from build123d import *

# Parameters (mm, degrees)
SKETCH1_W           = 50.8
SKETCH1_H           = 25.4
BOSS_EXTRUDE1_DEPTH = 660.4
SKETCH2_R           = 6.35
CUT_EXTRUDE1_DEPTH  = 254


with BuildPart() as part:
    # Sketch1 → Boss-Extrude1 (new body)
    with BuildSketch(Plane.XY):
        with Locations((25.4, 12.7)):
            Rectangle(SKETCH1_W, SKETCH1_H)
    extrude(amount=BOSS_EXTRUDE1_DEPTH)

    # Sketch2 → Cut-Extrude1 (cut)
    with BuildSketch(Plane(origin=(0, 25.4, 0), x_dir=(1, 0, 0), z_dir=(0, 1, 0))):
        with Locations((25.4, -63.5)):
            Circle(SKETCH2_R)
        with Locations((25.4, -571.5)):
            Circle(SKETCH2_R)
        with Locations((25.4, -330.2)):
            Circle(SKETCH2_R)
    extrude(amount=-CUT_EXTRUDE1_DEPTH, mode=Mode.SUBTRACT)


solid = part.part
Here's how the part is built. I have some questions about the finished solid (model axes, mm). Round coordinates to 2 decimals unless told otherwise and drop trailing zeros. Write each loop counter-clockwise with the first axis right and the second up, starting at its lowest first coordinate (ties: lowest second). Pieces come first, ordered by that corner, then holes.
1. I need wall thicknesses on L1, parallel to Z at x = 25.4, y = 16; L2, parallel to X at y = 5.5, z = 330.2. Which ranges of each line are inside material? Lowest first, please.
2. Suppose I cut it at B-B (z = 330.2). List the corners of the cut face in (x, y) for me, and give its area (3 significant figures).
3. Will this pin go through, and if not, where does the flat tip stop? pin 1 Ø4 at (x, y) = (34.5, 13.5) entering from -Z.
4. Suppose I cut it at A-A (x = 25.4). List the corners of the cut face in (y, z) for me, and give its area (3 significant figures).
5. If we mould it in two halves opening along X, with no side actions, what happens to faces 1 (the flat face through (50.8, 13, 326)), 2 (the flat face through (0, 13, 326)), 3 (the cylindrical face through (24.02, 12.88, 69.7))? For each: released by +X, released by -X, zero draft, split by the parting line, or undercut.
Answer sheet:
1. L1: z = 0 to 57.15, 69.85 to 323.85, 336.55 to 565.15, 577.85 to 660.4
1. L2: x = 0 to 19.05, 31.75 to 50.8
2. outline: (0, 0) - (19.05, 0) - (19.05, 25.4) - (0, 25.4) - close; (31.75, 0) - (50.8, 0) - (50.8, 25.4) - (31.75, 25.4) - close
2. area: 968 mm2
3. pin 1: stops at z = 0
4. outline: (0, 0) - (25.4, 0) - (25.4, 57.15) - (0, 57.15) - close; (0, 69.85) - (25.4, 69.85) - (25.4, 323.85) - (0, 323.85) - close; (0, 336.55) - (25.4, 336.55) - (25.4, 565.15) - (0, 565.15) - close; (0, 577.85) - (25.4, 577.85) - (25.4, 660.4) - (0, 660.4) - close
4. area: 15,800 mm2
5. face 1: released by +X
5. face 2: released by -X
5. face 3: undercut
